Work out the finished part from the listing and answer in its coordinate system (mm). A direction names the side the tool comes from. Round coordinates to 2 decimals unless told otherwise and drop trailing zeros. Write each loop counter-clockwise with the first axis right and the second up, starting at its lowest first coordinate (ties: lowest second). Pieces come first, ordered by that corner, then holes. Notation, with made-up numbers: M 50.5,-23 L 83.5,-23 A18 ccw 83.5,-6 Z; hole C -35,14 d1. An arc over 180 degrees is marked long. Answer in a Markdown table with one row per item.
```python
from build123d import *

# Parameters (mm, degrees)
CHAMFER1_SIZE = 0.25


with BuildPart() as part:
    # Sketch1 → Revolve1 (revolve)
    with BuildSketch(Plane.XY, mode=Mode.PRIVATE) as revolve1_sk:
        Polygon((-3, 0), (-3, 10), (-5, 10), (-5, 2), (-7, 2), (-7, 0), align=None)
    revolve(revolve1_sk.sketch.rotate(Axis((0, -356.558848917, 0), (0, 1, 0)), 180), axis=Axis((0, -356.558848917, 0), (0, 1, 0)))

    # Chamfer1
    chamfer1_edges = [part.edges().sort_by_distance(p)[0] for p in [
        (-7, 0, 0),
        (-7, 2, 0),
        (-5, 10, 0),
        (-3, 10, 0),
    ]]
    chamfer(chamfer1_edges, length=CHAMFER1_SIZE)


solid = part.part
```
1. Determine the mould class of faces 3 (the cylindrical face through (2.86, 4.94, -0.9)), 4 (the cylindrical face through (6.466, 0.99, 2.681)), 5 (the flat face through (-2, 10, 3)) for opening direction X: released by +X, released by -X, zero draft, split by the parting line, or undercut.
Calculated:
| item | result |
|---|---|
| face 3 | undercut |
| face 4 | split by the parting line |
| face 5 | zero draft |
2. The part is cut by section A-A (z = 0). Determine the outline of the cut face in (x, y).
Calculated:
| item | result |
|---|---|
| outline | M -7,0.25 L -6.75,0 L -3,0 L -3,9.75 L -3.25,10 L -4.75,10 L -5,9.75 L -5,2 L -6.75,2 L -7,1.75 Z; M 3,0 L 6.75,0 L 7,0.25 L 7,1.75 L 6.75,2 L 5,2 L 5,9.75 L 4.75,10 L 3.25,10 L 3,9.75 Z |
3. A tool of negligible diameter and unlimited length cuts with its end or side. For faces 1 (the flat face through (5, 2, 2)), 2 (the flat face through (3, 0, 1)), from which of +Z, -Z, +X, -X, +Y, -Y can it reach the whole face along a straight path? Write none if from no direction.
Calculated:
| item | result |
|---|---|
| face 1 | +Y |
| face 2 | +Z, -Z, +X, -X, -Y |
4. Consider line 1 along Z through (x, y) = (0, 5.75); line 2 along Z through (x, y) = (-2, 5.75). Determine where each line is inside the solid, lowest interval first. Write a range as from..to.
Calculated:
| item | result |
|---|---|
| line 1 | z = -5..-3, 3..5 |
| line 2 | z = -4.58..-2.24, 2.24..4.58 |
5. The part is cut by section B-B (x = 0). Determine the outline of the cut face in (y, z).
Calculated:
| item | result |
|---|---|
| outline | M 0,-6.75 L 0.25,-7 L 1.75,-7 L 2,-6.75 L 2,-5 L 9.75,-5 L 10,-4.75 L 10,-3.25 L 9.75,-3 L 0,-3 Z; M 0,3 L 9.75,3 L 10,3.25 L 10,4.75 L 9.75,5 L 2,5 L 2,6.75 L 1.75,7 L 0.25,7 L 0,6.75 Z |
6. Given pin 1 (6 mm diameter, centred on x = -3.5, y = 3, fed in from -Z); pin 2 (2 mm diameter, centred on x = -4, y = 6, fed in from -Z); pin 3 (2 mm diameter, centred on y = 4.5, z = 3, fed in from +X), each flat-ended and moving along its own axis, determine where each tip first touches the part or whether it passes through.
Calculated:
| item | result |
|---|---|
| pin 1 | stops at z = -6.96 |
| pin 2 | stops at z = -4 |
| pin 3 | stops at x = 4.58 |
7. The part is cut by section C-C (y = 2.25). Determine the outline of the cut face in (x, z).
Calculated:
| item | result |
|---|---|
| outline | C 0,0 d10; hole C 0,0 d6 |
